The listing builds one solid part. Answer for the finished solid, in the listing's coordinates (mm). A direction names the side the tool comes from. Round coordinates to 2 decimals unless told otherwise and drop trailing zeros. Answer in a Markdown table with one row per item. Add a question column.
```python
from build123d import *

# Parameters (mm, degrees)
F0_R     = 1.3
F1_DEPTH = 20
F2_DEPTH = 20
F3_DEPTH = 5


with BuildPart() as f1:
    # F0 (on Top) → F1 (new body)
    with BuildSketch(Plane.XY):
        with BuildLine():
            ThreePointArc((-7.18281, -3.909193), (-8.350454, -2.90793), (-7.573696, -1.580313))
            Line((-7.573696, -1.580313), (-7.573696, -1.5))
            Line((-7.573696, -1.5), (-12.162606, -1.5))
            add(Edge.make_bspline(
                [(-12.162606, -1.5), (-10.40903, -5.344737), (-3.038051, -6.305099)],
                knots=[0.232868, 0.232868, 0.232868, 1.325294, 1.325294, 1.325294], degree=2, weights=[1, 0.854498, 1]))
            Line((-3.038051, -6.305099), (-3.038051, -4.353841))
            Line((-3.038051, -4.353841), (-3.038051, -3.545245))
            Line((-3.038051, -3.545245), (-4.164727, -3.545245))
            ThreePointArc((-4.164727, -3.545245), (-4.346999, -3.582354), (-4.532958, -3.586717))
            Line((-4.532958, -3.586717), (-6.863885, -3.870381))
            ThreePointArc((-6.863885, -3.870381), (-7.022042, -3.900508), (-7.18281, -3.909193))
        make_face()
        with BuildLine():
            Line((-12.162606, -1.5), (-7.573696, -1.5))
            Line((-7.573696, -1.5), (-4.61644, -1.5))
            ThreePointArc((-4.61644, -1.5), (-4.464514, -1.488951), (-4.312587, -1.5))
            Line((-4.312587, -1.5), (0, -1.5))
            Line((0, -1.5), (1.807754, -2.1))
            Line((1.807754, -2.1), (11.829659, -2.1))
            add(Edge.make_bspline(
                [(11.829659, -2.1), (13.208327, 0), (11.829659, 2.1)],
                knots=[2.812614, 2.812614, 2.812614, 3.470572, 3.470572, 3.470572], degree=2, weights=[1, 0.946373, 1]))
            Line((11.829659, 2.1), (1.807754, 2.1))
            Line((1.807754, 2.1), (0, 1.5))
            Line((0, 1.5), (-12.162606, 1.5))
            add(Edge.make_bspline(
                [(-12.162606, 1.5), (-12.5, 0.76026), (-12.5, 0)],
                knots=[6.050317, 6.050317, 6.050317, 6.283185, 6.283185, 6.283185], degree=2, weights=[1, 0.993229, 1]))
            add(Edge.make_bspline(
                [(-12.5, 0), (-12.5, -0.76026), (-12.162606, -1.5)],
                knots=[0, 0, 0, 0.232868, 0.232868, 0.232868], degree=2, weights=[1, 0.993229, 1]))
        make_face()
        with Locations((4.42459, 0)):
            Circle(F0_R, mode=Mode.SUBTRACT)
        with BuildLine():
            add(Edge.make_bspline(
                [(11.829659, 2.1), (-2.165829, 23.418059), (-12.162606, 1.5)],
                knots=[3.470572, 3.470572, 3.470572, 6.050317, 6.050317, 6.050317], degree=2, weights=[1, 0.277243, 1]))
            Line((-12.162606, 1.5), (0, 1.5))
            Line((0, 1.5), (1.807754, 2.1))
            Line((1.807754, 2.1), (11.829659, 2.1))
        make_face()
        with BuildLine():
            Line((0, -1.5), (0, -6.5))
            add(Edge.make_bspline(
                [(0, -6.5), (8.941021, -6.5), (11.829659, -2.1)],
                knots=[1.570796, 1.570796, 1.570796, 2.812614, 2.812614, 2.812614], degree=2, weights=[1, 0.81335, 1]))
            Line((11.829659, -2.1), (1.807754, -2.1))
            Line((1.807754, -2.1), (0, -1.5))
        make_face()
    extrude(amount=-F1_DEPTH)

    # F0 (on Top) → F2 (join)
    with BuildSketch(Plane.XY):
        with BuildLine():
            ThreePointArc((-7.18281, -3.909193), (-8.350454, -2.90793), (-7.573696, -1.580313))
            Line((-7.573696, -1.580313), (-7.573696, -1.5))
            Line((-7.573696, -1.5), (-12.162606, -1.5))
            add(Edge.make_bspline(
                [(-12.162606, -1.5), (-10.40903, -5.344737), (-3.038051, -6.305099)],
                knots=[0.232868, 0.232868, 0.232868, 1.325294, 1.325294, 1.325294], degree=2, weights=[1, 0.854498, 1]))
            Line((-3.038051, -6.305099), (-3.038051, -4.353841))
            Line((-3.038051, -4.353841), (-3.038051, -3.545245))
            Line((-3.038051, -3.545245), (-4.164727, -3.545245))
            ThreePointArc((-4.164727, -3.545245), (-4.346999, -3.582354), (-4.532958, -3.586717))
            Line((-4.532958, -3.586717), (-6.863885, -3.870381))
            ThreePointArc((-6.863885, -3.870381), (-7.022042, -3.900508), (-7.18281, -3.909193))
        make_face()
        with BuildLine():
            add(Edge.make_bspline(
                [(11.829659, 2.1), (-2.165829, 23.418059), (-12.162606, 1.5)],
                knots=[3.470572, 3.470572, 3.470572, 6.050317, 6.050317, 6.050317], degree=2, weights=[1, 0.277243, 1]))
            Line((-12.162606, 1.5), (0, 1.5))
            Line((0, 1.5), (1.807754, 2.1))
            Line((1.807754, 2.1), (11.829659, 2.1))
        make_face()
        with BuildLine():
            Line((0, -1.5), (0, -6.5))
            add(Edge.make_bspline(
                [(0, -6.5), (8.941021, -6.5), (11.829659, -2.1)],
                knots=[1.570796, 1.570796, 1.570796, 2.812614, 2.812614, 2.812614], degree=2, weights=[1, 0.81335, 1]))
            Line((11.829659, -2.1), (1.807754, -2.1))
            Line((1.807754, -2.1), (0, -1.5))
        make_face()
    extrude(amount=F2_DEPTH)

    # F0 (on Top) → F3 (join)
    with BuildSketch(Plane.XY):
        with Locations((4.42459, 0)):
            Circle(F0_R)
    extrude(amount=-F3_DEPTH)


solid = f1.part
```
1. Straight lines are drawn through the part: line 1 along Y through (x, z) = (4, 6); line 2 along Z through (x, y) = (2.25, 0.75); line 3 along Y through (x, z) = (8.25, 3.5). For each, find the intervals that lie inside material, in ascending order.
2. For faces 4 (the flat face through (-6, -1.5, -10)), 5 (the flat face through (0.9, -1.8, 9.9)), 6 (the flat face through (-3.038, -5, 0)), 7 (the flat face through (4, 0, -5)), 8 (the flat face through (-10, -1.5, 10)), determine the directions among +Z, -Z, +X, -X, +Y, -Y from which every point of the face is accessible in a straight line to the end or side of a thin tool.
3. Each of these flat-tipped pins is pushed along its axis until it touches: pin 1 (1.6 mm diameter, centred on x = 4.42, y = 0, fed in from +Z); pin 2 (3 mm diameter, centred on y = -5.5, z = -3, fed in from +X); pin 3 (5 mm diameter, centred on x = -10, z = 7, fed in from +Y). Where does it stop, or does it pass through?
4. The mould has two halves that part along X. Classify faces 1 (the flat face through (0, 0, -20)), 2 (the flat face through (0.9, 1.8, 9.9)), 3 (the flat face through (0, -4, 0)): released by +X, released by -X, zero draft, split by the parting line, or undercut.
5. The part is cut by section A-A (z = 17). Give the number of separate pieces and of enclosed holes in the cut face, then the cut area to 3 significant figures.
Report:
| question | item | result |
|---|---|---|
| 1 | line 1 | y = -6.16 to -2.1, 2.1 to 6.16 |
| 1 | line 2 | z = -20 to 0 |
| 1 | line 3 | y = -4.88 to -2.1, 2.1 to 4.88 |
| 2 | face 4 | +Z, -Z |
| 2 | face 5 | +Z, +X |
| 2 | face 6 | +Z, -Z, -Y |
| 2 | face 7 | -Z |
| 2 | face 8 | +Z, +X, -X |
| 3 | pin 1 | stops at z = 0 |
| 3 | pin 2 | stops at x = 9.85 |
| 3 | pin 3 | stops at y = 5.2 |
| 4 | face 1 | zero draft |
| 4 | face 2 | released by +X |
| 4 | face 3 | undercut |
| 5 | separate pieces | 3 |
| 5 | enclosed holes | 0 |
| 5 | area | 141 mm^2 |
